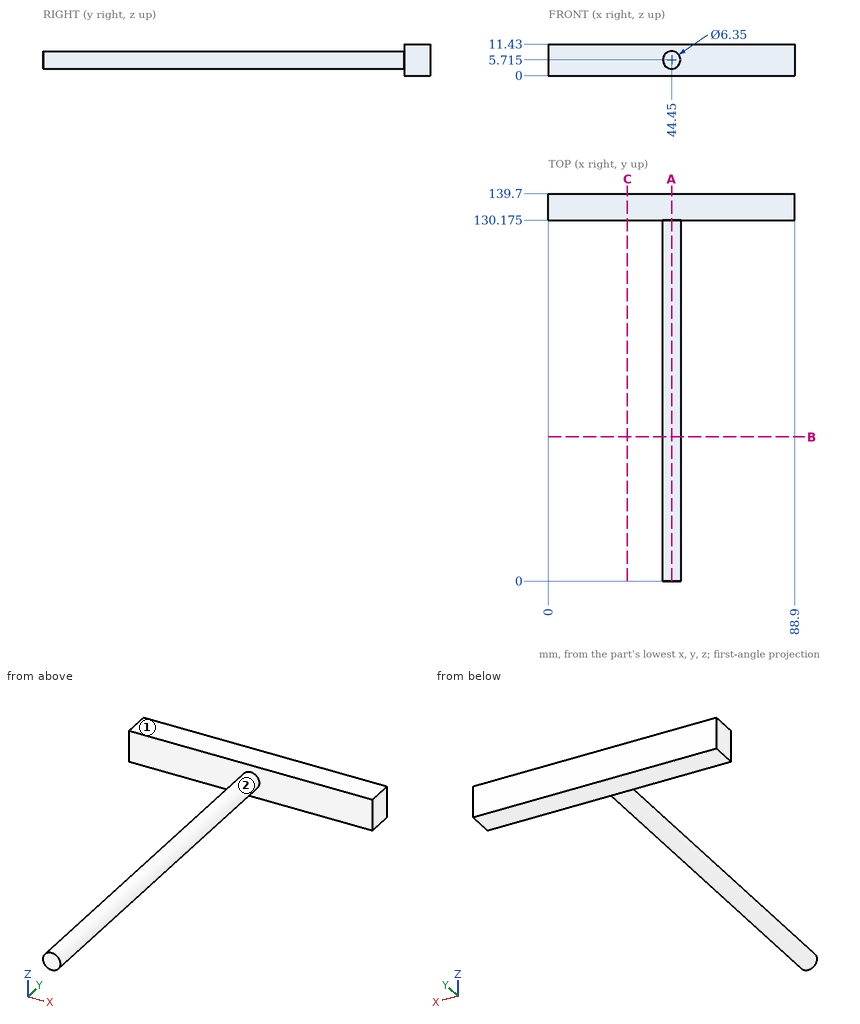
Verification items for this drawing (mm, ordinates from the low corner). A direction names the side the tool comes from. Round coordinates to 2 decimals unless told otherwise and drop trailing zeros. Write each loop counter-clockwise with the first axis right and the second up, starting at its lowest first coordinate (ties: lowest second). Pieces come first, ordered by that corner, then holes. Notation, with made-up numbers: M 7,45.25 L 16,45.25 A23 cw 16,55.25 Z; hole C 33.5,-19 d3. An arc over 180 degrees is marked long. Write item = value, one per line. Start each with the question number.
1. Section check B-B, the plane y = 52. Record the cut outline in (x, z) (3 decimals), then the cut area to 3 significant figures.
2. Gauge pin test, flat ends, axial feed: pin 1 (1 mm diameter, centred on y = 91.5, z = 6.5, fed in from +X); pin 2 (3 mm diameter, centred on y = 114.5, z = 8.5, fed in from -X); pin 3 (4 mm diameter, centred on x = 44.5, y = 24.5, fed in from +Z). Record the tip position at first contact, or that the pin passes through.
3. Section check C-C, the plane x = 28.5. Record the cut outline in (y, z) (3 decimals).
4. Section check A-A, the plane x = 44.45. Record the cut outline in (y, z) (3 decimals), then the cut area to 3 significant figures.
5. Tool access check on the marked faces 1 and 2. Record the directions out of +Z, -Z, +X, -X, +Y, -Y that give a thin tool (end or side, any length) a straight path to the whole face; none if there is none.
6. Scan lines: line 1 (Y direction, x = 19, z = 1.25) (3 decimals); line 2 (Z direction, x = 44, y = 114); line 3 (X direction, y = 60.5, z = 5.5). Record each from-to range of solid material in increasing order. Write a range as [from, to].
Results found:
q1.outline = C 44.45,5.715 d6.35
q1.area = 31.7 mm^2
q2.pin_1 = 47.61
q2.pin_2 = 41.55
q2.pin_3 = 8.89
q3.outline = M 130.175,0 L 139.7,0 L 139.7,11.43 L 130.175,11.43 Z
q4.outline = M 0,2.54 L 130.175,2.54 L 130.175,0 L 139.7,0 L 139.7,11.43 L 130.175,11.43 L 130.175,8.89 L 0,8.89 Z
q4.area = 935 mm^2
q5.face_1 = +Z, +X, -X, +Y, -Y
q5.face_2 = -Y
q6.line_1 = [130.175, 139.7]
q6.line_2 = [2.57, 8.86]
q6.line_3 = [41.28, 47.62]
